For this review, take the finished solid that the model builds, in its own axes (mm). Face numbers are marked on the shaded views. Coordinates: 2 decimals unless noted, no trailing zeros. Loops run counter-clockwise (first coordinate to the right, second up) from the corner with the lowest first, then second, coordinate; pieces in that order, holes last. Notation, with made-up numbers: (62.5, -11.5) - (118.5, -11.5) arc R29 cw to (118.5, 17.5) - close; hole circle Ø7 at (-3.75, 40). An arc over 180 degrees is marked (long way). One line per item, written item: value. Start each with the question number.
1. Insertion check: pin 1 (2.5 mm diameter, centred on y = -2, z = 0, fed in from -X); pin 2 (2.5 mm diameter, centred on y = -2.5, z = -13, fed in from +X); pin 3 (2.5 mm diameter, centred on x = 24.5, y = -3.5, fed in from -Z). Each pin has a flat end and moves straight along its axis. Give the tip position at first contact, or say it passes through.
2. Take a section at B-B, the plane y = -2.05. State the section outline as (x, z) points.
3. Take a section at A-A, the plane z = -8. State the section outline as (x, y) points, and give its area (3 significant figures).
4. Take a section at D-D, the plane x = -11.5. State the section outline as (y, z) points.
5. To check wall thickness, follow line 1 (X direction, y = -3.4, z = 14); line 2 (X direction, y = -3.5, z = -8); line 3 (X direction, y = -1, z = -4). State the ranges of each line that lie inside material, in increasing order. Write a range as from..to.
6. The part is to be moulded in two halves that separate along X. For the marked faces 1, 2 and 3, say which applies: released by +X, released by -X, zero draft, split by the parting line, or undercut.
7. Take a section at C-C, the plane z = 3. State the section outline as (x, y) points, and give its area (3 significant figures).
```python
from build123d import *

# Parameters (mm, degrees)
F2_DEPTH = 5


with BuildPart() as f2:
    # F0 (on Front) → F2 (new body)
    with BuildSketch(Plane.XZ):
        with BuildLine():
            Line((23, 20), (23, 5))
            Line((23, 5), (26, 5))
            Line((26, 5), (26, 20))
            ThreePointArc((26, 20), (13, 33), (0, 20))
            Line((0, 20), (0, 0))
            Line((0, 0), (3, 0))
            Line((3, 0), (3, 20))
            ThreePointArc((3, 20), (13, 30), (23, 20))
        make_face()
        with BuildLine():
            Line((3, -20), (3, 0))
            Line((3, 0), (0, 0))
            Line((0, 0), (0, -20))
            ThreePointArc((0, -20), (-11.5, -31.5), (-23, -20))
            Line((-23, -20), (-23, -5))
            Line((-23, -5), (-26, -5))
            Line((-26, -5), (-26, -20))
            ThreePointArc((-26, -20), (-11.5, -34.5), (3, -20))
        make_face()
    extrude(amount=F2_DEPTH)


solid = f2.part
```
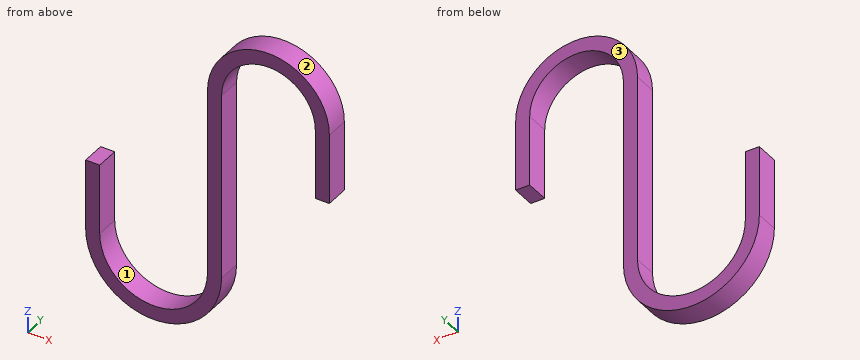
Solutions:
1. pin 1: x = 0
1. pin 2: x = 3
1. pin 3: z = 5
2. outline: (-26, -20) arc R14.5 ccw to (3, -20) - (3, 20) arc R10 cw to (23, 20) - (23, 5) - (26, 5) - (26, 20) arc R13 ccw to (0, 20) - (0, -20) arc R11.5 cw to (-23, -20) - (-23, -5) - (-26, -5) - close
3. outline: (-26, -5) - (-23, -5) - (-23, 0) - (-26, 0) - close; (0, -5) - (3, -5) - (3, 0) - (0, 0) - close
3. area: 30.0 mm2
4. outline: (-5, -34.5) - (0, -34.5) - (0, -31.5) - (-5, -31.5) - close
5. line 1: 0..3, 23..26
5. line 2: -26..-23, 0..3
5. line 3: 0..3
6. face 1: undercut
6. face 2: split by the parting line
6. face 3: zero draft
7. outline: (0, -5) - (3, -5) - (3, 0) - (0, 0) - close
7. area: 15.0 mm2
